Could you check a few things on this model? Use its own coordinates, in mm. A direction names the side the tool comes from. Give positions to 0.01 mm unless a question says otherwise; leave off trailing zeros. Write each loop counter-clockwise with the first axis right and the second up, starting at its lowest first coordinate (ties: lowest second). Pieces come first, ordered by that corner, then holes. Notation, with made-up numbers: (48, -24.75) - (101, -24.75) arc R26 ccw to (101, 8.25) - close; hole circle Ø7 at (-2.75, 64.25). An arc over 180 degrees is marked (long way). Answer in a Markdown table with one row per item.
Autodesk Inventor part; units mm, degrees
ref_plane "YZ Plane" through (0, 0, 0) normal (1, 0, 0) x (0, 1, 0)
ref_plane "XZ Plane" through (0, 0, 0) normal (0, 1, 0) x (-1, 0, 0)
ref_plane "XY Plane" through (0, 0, 0) normal (0, 0, 1) x (1, 0, 0)
sketch "Sketch1" plane through (0, 0, 0) normal (0, 0, 1) x (1, 0, 0)
  line L0 (-2, 10.5) -> (0, 10.5)
  line L1 (0, 10.5) -> (0, 19)
  line L2 (0, 19) -> (8.5, 19)
  line L3 (8.5, 19) -> (8.5, 8)
  line L4 (8.5, 8) -> (-2, 8)
  line L5 (-2, 8) -> (-2, 10.5)
  line L6 (-3.774, 0) -> (9.2238, 0)
  point P0 (0, 0)
  dimension "d0" = 38
  dimension "d1" = 8.5
  dimension "d2" = 10.5
  dimension "d3" = 16
  dimension "d4" = 21
revolve "Revolution1" add sketch "Sketch1" angle 360 about axis through (-3.774, 0, 0) along (1, 0, 0)
sketch "Sketch2" plane through (8.5, 0, 0) normal (1, 0, 0) x (0, 0, -1)
  line L0 (14, -19) -> (-14, -19)
  line L1 (-14, -19) -> (-14, 19)
  line L2 (-14, 19) -> (14, 19)
  line L3 (14, 19) -> (14, -19)
  line L4 (14, -19) -> (-14, 19) construction
  line L5 (-14, -19) -> (14, 19) construction
  circle A0 centre (0, 0) radius 19
  dimension "d6" = 28
extrude "Extrusion1" cut sketch "Sketch2" against normal blind 10 contours L0 A0 L3 | L0 L1 A0 | A0 L1 L3 | A0 L2 L3 | L1 L2 A0 keep common part
sketch "Sketch3" plane through (8.5, -12.8452, 14) normal (1, 0, 0) x (0, 0, -1)
  point P0 (14, 12.8452)
  point P1 (14, -2.1548)
  point P2 (14, 27.8452)
  dimension "d9" = 30
  dimension "d10" = 15
hole "Hole1" at (8.5, -15, 0) at (8.5, 15, 0) direction (-1, 0, 0) diameter 3.5 end through all counterbore diameter 6.5 counterbore depth 4
properties part number "Endpuffer" material "PMMA Plastic"
1) If I drill on line 1 (Y direction, x = 0.75, z = 1.25); line 2 (Y direction, x = 5.5, z = -0.5); line 3 (Z direction, x = 4.75, y = 0), over which ranges is the centre line in solid material (lowest first)?
Check values:
| item | result |
|---|---|
| line 1 | y = -18.96 to -16.22, -13.78 to -7.9, 7.9 to 13.78, 16.22 to 18.96 |
| line 2 | y = -18.99 to -18.21, -11.79 to -7.98, 7.98 to 11.79, 18.21 to 18.99 |
| line 3 | z = -14 to -8, 8 to 14 |
2) Imagine slicing it at B-B (z = 0). List the corners of the cut face in (x, y) for me, then the cut area to 3 significant figures.
Check values:
| item | result |
|---|---|
| outline | (-1.5, -10.5) - (0, -10.5) - (0, -13.25) - (4.5, -13.25) - (4.5, -11.75) - (8.5, -11.75) - (8.5, -8) - (-1.5, -8) - close; (-1.5, 8) - (8.5, 8) - (8.5, 11.75) - (4.5, 11.75) - (4.5, 13.25) - (0, 13.25) - (0, 10.5) - (-1.5, 10.5) - close; (0, -19) - (8.5, -19) - (8.5, -18.25) - (4.5, -18.25) - (4.5, -16.75) - (0, -16.75) - close; (0, 16.75) - (4.5, 16.75) - (4.5, 18.25) - (8.5, 18.25) - (8.5, 19) - (0, 19) - close |
| area | 111 mm2 |
3) On a 3-axis mill with a long thin cutter (end or side, diameter ignored), from which of +Z, -Z, +X, -X, +Y, -Y can I reach the whole of each face in a straight line? I mean faces 1 (the face through (0, -4, 10)), 2 (the face through (4, -19, 0)), 3 (the face through (6.472, 11.778, 0.423)). Say none if no direction works.
Check values:
| item | result |
|---|---|
| face 1 | -X |
| face 2 | +X, -X, -Y |
| face 3 | +X |
4) Will these pins go through, and if not, where does the flat tip stop? P1, Ø1, axis at x = 5.5, z = 8, coming from the +Y side; P2, Ø5, axis at y = -15, z = 0, coming from the -X side; P3, Ø2, axis at y = -14, z = 0, coming from the +X side.
Check values:
| item | result |
|---|---|
| P1 | stops at y = 17.46 |
| P2 | stops at x = 0 |
| P3 | stops at x = 4.5 |
5) We'd pull the mould along Z, two halves only. Please class faces 4 (the face through (8.5, 8.2, 0.2)), 5 (the face through (2.218, -16.735, 0.228)), 6 (the face through (-0.7, 10, 3.2)): +Z half, -Z half, draft (parallel to the pull), parting line (faces both ways), or undercut.
Check values:
| item | result |
|---|---|
| face 4 | draft |
| face 5 | undercut |
| face 6 | parting line |
6) Imagine slicing it at C-C (x = 0.75). List the corners of the cut face in (y, z) for me.
Check values:
| item | result |
|---|---|
| outline | (-12.85, -14) - (12.85, -14) arc R19 ccw to (12.85, 14) - (-12.85, 14) arc R19 ccw to start; hole circle Ø3.5 at (-15, 0); hole circle Ø16 at (0, 0); hole circle Ø3.5 at (15, 0) |
7) Imagine slicing it at A-A (y = 0). List the corners of the cut face in (x, z) for me.
Check values:
| item | result |
|---|---|
| outline | (-1.5, -10.5) - (0, -10.5) - (0, -14) - (8.5, -14) - (8.5, -8) - (-1.5, -8) - close; (-1.5, 8) - (8.5, 8) - (8.5, 14) - (0, 14) - (0, 10.5) - (-1.5, 10.5) - close |
8) Imagine slicing it at D-D (z = 7.25). List the corners of the cut face in (x, y) for me, then the cut area to 3 significant figures.
Check values:
| item | result |
|---|---|
| outline | (-1.5, -7.6) - (0, -7.6) - (0, -17.56) - (8.5, -17.56) - (8.5, -3.38) - (-1.5, -3.38) - close; (-1.5, 3.38) - (8.5, 3.38) - (8.5, 17.56) - (0, 17.56) - (0, 7.6) - (-1.5, 7.6) - close |
| area | 254 mm2 |
